```python
from build123d import *

# Parameters (mm, degrees)
SKETCH1_R           = 6.35
SKETCH1_R_2         = 3.175
SKETCH1_W           = 26.67
SKETCH1_H           = 31.75
BOSS_EXTRUDE1_DEPTH = 6.35
BOSS_EXTRUDE2_DEPTH = 19.05
FILLET1_R           = 50.8


with BuildPart() as part:
    # Sketch1 → Boss-Extrude1 (new body)
    with BuildSketch(Plane(origin=(0, 0, 0), x_dir=(1, 0, 0), z_dir=(0, 1, 0))):
        Polygon((-76.2, 88.9), (76.2, 88.9), (76.2, -50.8), (38.1, -88.9), (-38.1, -88.9), (-76.2, -50.8), align=None)
        with Locations((52.07, 25.4)):
            Circle(SKETCH1_R, mode=Mode.SUBTRACT)
        with Locations((-25.4, -50.8)):
            Circle(SKETCH1_R, mode=Mode.SUBTRACT)
        with Locations((25.4, -50.8)):
            Circle(SKETCH1_R, mode=Mode.SUBTRACT)
        with Locations((0, -76.2)):
            Circle(SKETCH1_R_2, mode=Mode.SUBTRACT)
        with Locations((0, 76.2)):
            Circle(SKETCH1_R_2, mode=Mode.SUBTRACT)
        with Locations((-52.07, 25.4)):
            Circle(SKETCH1_R, mode=Mode.SUBTRACT)
        with Locations((13.335, 25.4)):
            Circle(SKETCH1_R_2, mode=Mode.SUBTRACT)
        with Locations((-13.335, 25.4)):
            Rectangle(SKETCH1_W, SKETCH1_H, mode=Mode.SUBTRACT)
    extrude(amount=BOSS_EXTRUDE1_DEPTH)

    # Sketch2 → Boss-Extrude2 (add)
    with BuildSketch(Plane(origin=(0, 0, 0), x_dir=(1, 0, 0), z_dir=(0, 1, 0))):
        Polygon((-76.2, 88.9), (-76.2, -50.8), (-38.1, -88.9), (38.1, -88.9), (76.2, -50.8), (76.2, 88.9), align=None)
        Polygon((-69.85, 82.55), (-69.85, -48.169743879), (-35.469743879, -82.55), (35.469743879, -82.55), (69.85, -48.169743879), (69.85, 82.55), align=None, mode=Mode.SUBTRACT)
    extrude(amount=BOSS_EXTRUDE2_DEPTH)

    # Fillet1
    fillet1_edges = [part.edges().sort_by_distance(p)[0] for p in [
        (76.2, 9.525, 50.8),
        (38.1, 9.525, 88.9),
        (-38.1, 9.525, 88.9),
        (-76.2, 9.525, 50.8),
    ]]
    fillet(fillet1_edges, radius=FILLET1_R)


solid = part.part
```
Source: CAD feature listing. Evaluate the final solid. Frame: model axes, mm. A direction names the side the tool comes from. Round coordinates to 2 decimals unless told otherwise and drop trailing zeros. Loops run counter-clockwise (first coordinate to the right, second up) from the corner with the lowest first, then second, coordinate; pieces in that order, holes last. Notation, with made-up numbers: M 49.5,12.25 L 64.5,12.25 A28 ccw 64.5,32.25 Z; hole C 53,23.5 d11. An arc over 180 degrees is marked long. Put each result on its own line as item: value.
(1) Section C-C, the plane y = 9. Return loops of the section in (x, z), and give its area (3 significant figures).
Solutions:
outline: M -76.2,-88.9 L 76.2,-88.9 L 76.2,29.76 A50.8 ccw 61.32,65.68 L 52.98,74.02 A50.8 ccw 17.06,88.9 L -17.06,88.9 A50.8 ccw -52.98,74.02 L -61.32,65.68 A50.8 ccw -76.2,29.76 Z; hole M -69.85,-82.55 L 69.85,-82.55 L 69.85,48.17 L 35.47,82.55 L -35.47,82.55 L -69.85,48.17 Z
area: 3,540 mm²
(2) Section B-B, the plane x = 6.5. Return loops of the section in (y, z), and give its area (3 significant figures).
Solutions:
outline: M 0,-88.9 L 19.05,-88.9 L 19.05,-82.55 L 6.35,-82.55 L 6.35,82.55 L 19.05,82.55 L 19.05,88.9 L 0,88.9 Z
area: 1,290 mm²
(3) Section A-A, the plane z = -76.2. Return loops of the section in (x, y) (3 decimals), and give its area (3 significant figures).
Solutions:
outline: M -76.2,0 L -3.175,0 L -3.175,6.35 L -69.85,6.35 L -69.85,19.05 L -76.2,19.05 Z; M 3.175,0 L 76.2,0 L 76.2,19.05 L 69.85,19.05 L 69.85,6.35 L 3.175,6.35 Z
area: 1,090 mm²
(4) Access query for faces 1 (the face through (0, 19.05, -86)), 2 (the face through (69.85, 13, -16)), 3 (the face through (0, 3, -25)). Directions: +Z, -Z, +X, -X, +Y, -Y. A direction counts if a zero-diameter tool reaches every point of the face in a straight line with its end or side. Return the directions, or none.
Solutions:
face 1: +Z, -Z, +X, -X, +Y
face 2: +Y
face 3: +Y, -Y
(5) Ray query, line 1 (X direction, y = 1.75, z = -25.4); line 2 (X direction, y = 7.75, z = -47); line 3 (Z direction, x = -12.5, y = 11.25). Return the intervals inside material, ascending. Write a range as [from, to].
Solutions:
line 1: [-76.2, -58.42], [-45.72, -26.67], [0, 10.16], [16.51, 45.72], [58.42, 76.2]
line 2: [-76.2, -69.85], [69.85, 76.2]
line 3: [-88.9, -82.55], [82.55, 88.9]
(6) First-contact query: pin 1 (10 mm diameter, centred on x = 25, y = 3.5, fed in from +Z); pin 2 (5 mm diameter, centred on x = 0, z = 76.2, fed in from +Y); pin 3 (4 mm diameter, centred on x = -45.5, z = -32, fed in from +Y). Flat tips, straight axial feed; report the tip coordinate or a pass-through.
Solutions:
pin 1: z = 88.81
pin 2: through
pin 3: y = 6.35
(7) Section D-D, the plane z = -25.4. Return loops of the section in (x, y).
Solutions:
outline: M -76.2,0 L -58.42,0 L -58.42,6.35 L -69.85,6.35 L -69.85,19.05 L -76.2,19.05 Z; M -45.72,0 L -26.67,0 L -26.67,6.35 L -45.72,6.35 Z; M 0,0 L 10.16,0 L 10.16,6.35 L 0,6.35 Z; M 16.51,0 L 45.72,0 L 45.72,6.35 L 16.51,6.35 Z; M 58.42,0 L 76.2,0 L 76.2,19.05 L 69.85,19.05 L 69.85,6.35 L 58.42,6.35 Z
(8) Pull-direction query (Z, two-part tool) for faces 4 (the face through (-1, 9, -88.9)), 5 (the face through (0, 9, 88.9)), 6 (the face through (0, 13, 82.55)), 7 (the face through (76.2, 9, -30)); classes: released by +Z, released by -Z, zero draft, split by the parting line, or undercut.
Solutions:
face 4: released by -Z
face 5: released by +Z
face 6: undercut
face 7: zero draft
